The model under review builds one solid part; all positions refer to its coordinate system, in mm. A direction names the side the tool comes from. Give positions to 0.01 mm unless a question says otherwise; leave off trailing zeros. Order: outer loops, then holes, each group sorted by start corner. A loop starts at its lowest first (then second) coordinate and runs counter-clockwise, first axis right, second up. Notation, with made-up numbers: (-29, 77.25) - (11, 77.25) arc R32 ccw to (11, 116.25) - close; hole circle Ø4 at (37.25, -9). An arc over 180 degrees is marked (long way). Write item = value, one per line. Start each with the question number.
1. We need section A-A, the plane z = 7.75. Give the boundary of the cut face in (x, y).
2. Machinability: for faces 1 (the flat face through (0, 0, 20)), 2 (the cylindrical face through (-8.256, -21.43, 8.573)), which of the approach directions +Z, -Z, +X, -X, +Y, -Y give a long, thin tool a straight path to every point of the face, cutting with its end or side? Answer none if there is none.
3. For P1, Ø10, axis at x = 8, z = 13, coming from the -Y side; P2, Ø12, axis at x = -10.5, z = 10.5, coming from the -Y side, all flat-tipped, find the tip position at first contact; note any pin that passes through.
4. We need section B-B, the plane x = 3.5. Give the boundary of the cut face in (y, z), and give its area (3 significant figures).
5. Wall thickness on probe 1 along Y at (x, z) = (-12, 16.5); probe 2 along X at (y, z) = (-18.5, 6.25); probe 3 along Z at (x, y) = (-10.5, -18.5): over which ranges is each line inside the solid? List them lowest first.
6. We need section C-C, the plane z = 17.5. Give the boundary of the cut face in (x, y), and give its area (3 significant figures).
from build123d import *

# Parameters (mm, degrees)
SKETCH1_W           = 33
SKETCH1_H           = 33
BOSS_EXTRUDE1_DEPTH = 20
SKETCH2_R           = 3.018628297
BOSS_EXTRUDE2_DEPTH = 10


with BuildPart() as part:
    # Sketch1 → Boss-Extrude1 (new body)
    with BuildSketch(Plane.XY):
        Rectangle(SKETCH1_W, SKETCH1_H)
    extrude(amount=BOSS_EXTRUDE1_DEPTH)

    # Sketch2 → Boss-Extrude2 (add)
    with BuildSketch(Plane.XZ.offset(16.5)):
        with Locations(Location((-10.934193972, 7.179785009, 0), (0, 0, 90))):
            Circle(SKETCH2_R)
    extrude(amount=BOSS_EXTRUDE2_DEPTH)


solid = part.part
Model answer:
q1.outline = (-16.5, -16.5) - (-13.9, -16.5) - (-13.9, -26.5) - (-7.97, -26.5) - (-7.97, -16.5) - (16.5, -16.5) - (16.5, 16.5) - (-16.5, 16.5) - close
q2.face_1 = +Z, +X, -X, +Y, -Y
q2.face_2 = -Y
q3.P1 = -16.5
q3.P2 = -26.5
q4.outline = (-16.5, 0) - (16.5, 0) - (16.5, 20) - (-16.5, 20) - close
q4.area = 660 mm2
q5.probe_1 = -16.5 to 16.5
q5.probe_2 = -13.81 to -8.06
q5.probe_3 = 4.19 to 10.17
q6.outline = (-16.5, -16.5) - (16.5, -16.5) - (16.5, 16.5) - (-16.5, 16.5) - close
q6.area = 1,090 mm2
